Part print with two shaded views. Sizes in mm from the minimum x, y, z corner. Round coordinates to 2 decimals unless told otherwise and drop trailing zeros. Loops run counter-clockwise (first coordinate to the right, second up) from the corner with the lowest first, then second, coordinate; pieces in that order, holes last. Notation, with made-up numbers: (3, 53) - (44, 53) arc R21 cw to (44, 81) - close; hole circle Ø10 at (17.5, -37). An arc over 180 degrees is marked (long way). One line per question, with ' | ' between items.
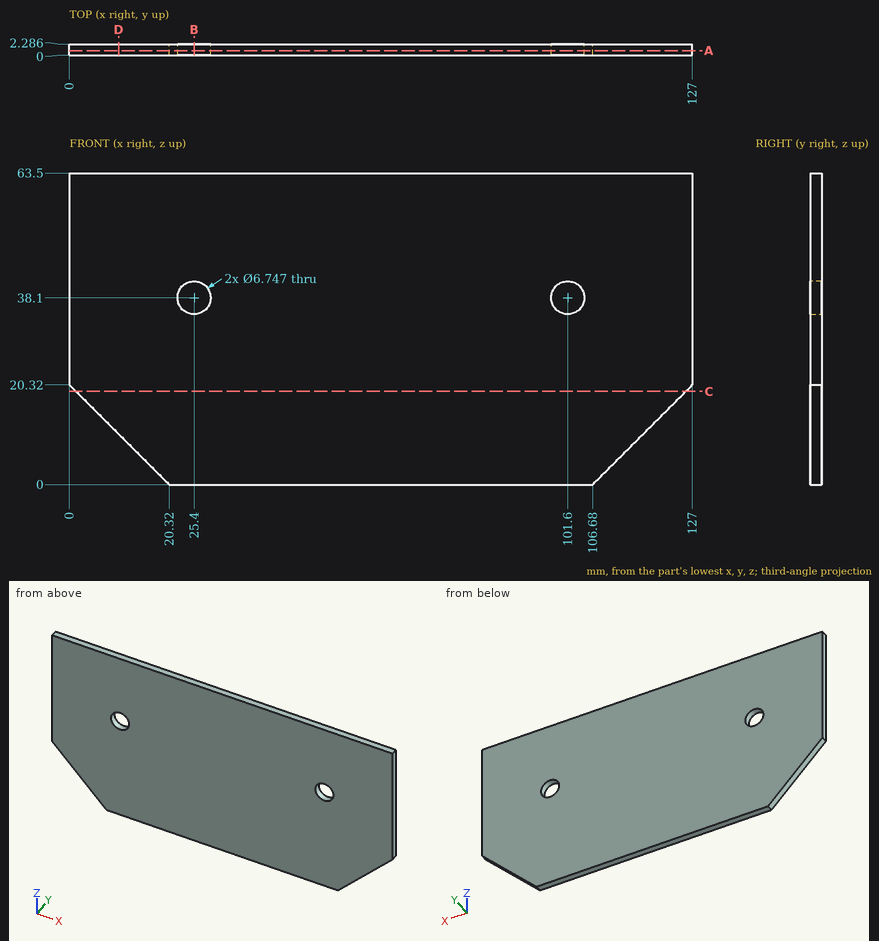
(1) Drop a flat-ended pin along its axis: P1, Ø8, axis at x = 101.6, z = 38.1, coming from the -Y side. Give the stop position or say it passes through.
Results found:
P1: stops at y = 0
(2) Cut at A-A, the plane y = 0.95. Write the cut outline in (x, z), then the cut area to 3 significant figures.
Results found:
outline: (0, 20.32) - (20.32, 0) - (106.68, 0) - (127, 20.32) - (127, 63.5) - (0, 63.5) - close; hole circle Ø6.75 at (25.4, 38.1); hole circle Ø6.75 at (101.6, 38.1) | area: 7,580 mm²
(3) Cut at D-D, the plane x = 10. Write the cut outline in (y, z).
Results found:
outline: (0, 10.32) - (2.29, 10.32) - (2.29, 63.5) - (0, 63.5) - close
(4) Cut at C-C, the plane z = 19. Write the cut outline in (x, y), then the cut area to 3 significant figures.
Results found:
outline: (1.32, 0) - (125.68, 0) - (125.68, 2.29) - (1.32, 2.29) - close | area: 284 mm²
(5) Probe L1, parallel to X at y = 0.5, z = 38.1; L2, parallel to X at y = 0.3, z = 37.5; L3, parallel to Z at x = 13, y = 0.1. List the from-to ranges inside material, lowest first.
Results found:
L1: x = 0 to 22.03, 28.77 to 98.23, 104.97 to 127 | L2: x = 0 to 22.08, 28.72 to 98.28, 104.92 to 127 | L3: z = 7.32 to 63.5
(6) Cut at B-B, the plane x = 25.4. Write the cut outline in (y, z), then the cut area to 3 significant figures.
Results found:
outline: (0, 0) - (2.29, 0) - (2.29, 34.73) - (0, 34.73) - close; (0, 41.47) - (2.29, 41.47) - (2.29, 63.5) - (0, 63.5) - close | area: 130 mm²
